Build history of the part. All positions in model axes, mm. A direction names the side the tool comes from. Give positions to 0.01 mm unless a question says otherwise; leave off trailing zeros. Order: outer loops, then holes, each group sorted by start corner. A loop starts at its lowest first (then second) coordinate and runs counter-clockwise, first axis right, second up. Notation, with made-up numbers: (54.5, 87) - (72.5, 87) arc R9 ccw to (72.5, 92) - close; hole circle Ø2 at (1.5, 15). An arc over 180 degrees is marked (long way). Write each question's results on one line, items separated by ' | '. Start each with the question number.
1) Two-plate mould, pull along Y, no slides. Class faces 4 (the face through (0, 46.189, 1)), 5 (the face through (21.09, -36.31, 68.49)), 6 (the face through (0, -26.707, 16)): +Y half, -Y half, draft (parallel to the pull), parting line (faces both ways), or undercut.
2) Tool access for faces 1 (the face through (-21.18, 0.59, -26.29)), 2 (the face through (21.18, 0.59, -26.29)), 3 (the face through (29.472, 37, -1)): list every direction of +Z, -Z, +X, -X, +Y, -Y with a clear straight run to the whole face (end or side of a thin tool).
3) Drop flat-ended pins along their axis: pin 1 Ø10 at (x, y) = (-6, -33) entering from -Z; pin 2 Ø4 at (x, y) = (-19.5, 24) entering from -Z; pin 3 Ø5 at (x, y) = (7.5, 2.5) entering from -Z. Give the stop position or say it passes through.
4) Drill centre lines: line 1 along Y through (x, z) = (-25, 37); line 2 along Z through (x, y) = (-3.5, -29); line 3 along Z through (x, y) = (-7, -34). Where is each one in solid material? Low to high. Write a range as from..to.
5) Cut at C-C on z = 59. List the corners of the cut face in (x, y).
6) Cut at A-A on y = 33. List the corners of the cut face in (x, z).
7) Cut at D-D on x = -7.5. List the corners of the cut face in (y, z).
8) Cut at B-B on z = -9.5. List the corners of the cut face in (x, y).
from build123d import *

# Parameters (mm, degrees)
F0_W        = 58.9435696602
F0_H        = 155.2014648914
F4_DEPTH    = 46.1890073493
F5_W        = 53.8340881467
F5_H        = 92.8563177586
F1_DEPTH    = 58.9445696602
F2_T1_DEPTH = 168.3050352459
F2_T3_DEPTH = 168.726075006
F2_T5_DEPTH = 241.6216065486
F3_T1_DEPTH = 53.8340881467
F6_R        = 13.164421927
F6_R_2      = 14.3764863779
F7_DEPTH    = 92.3790146986


# Not quite as in the source:
# - a fillet or chamfer that OpenCascade refuses, or shapes differently, is made with other operations: its cross-section is extruded or revolved along the edge and cut away or added


with BuildPart() as f4:
    # F0 (on Front) → F4 (new body, symmetric)
    with BuildSketch(Plane.XZ):
        Rectangle(F0_W, F0_H)
    extrude(amount=F4_DEPTH, both=True)

    # F5 (on face) → F1 (cut, through all)
    with BuildSketch(Plane.YZ.offset(29.4717848301)):
        with Locations((0.2105198801, 31.1725735664)):
            Rectangle(F5_W, F5_H)
    extrude(amount=-F1_DEPTH, mode=Mode.SUBTRACT)

    # F2: fillet of radius 29.84871837 on 6 edges, made by hand

    # F2_s2 → F2_t1 (cut)
    with BuildSketch(Plane.XZ.offset(-120.8108032743)):
        with BuildLine():
            ThreePointArc((29.4717848301, 47.7520140757), (20.7292976292, 68.8582452449), (-0.3769335399, 77.6007324457))
            Line((-0.3769335399, 77.6007324457), (29.4717848301, 77.6007324457))
            Line((29.4717848301, 77.6007324457), (29.4717848301, 47.7520140757))
        make_face()
        with BuildLine():
            ThreePointArc((-29.4717848301, 47.7520140757), (-20.7292976292, 68.8582452449), (0.3769335399, 77.6007324457))
            Line((0.3769335399, 77.6007324457), (-29.4717848301, 77.6007324457))
            Line((-29.4717848301, 77.6007324457), (-29.4717848301, 47.7520140757))
        make_face()
    extrude(amount=F2_T1_DEPTH, mode=Mode.SUBTRACT)

    # F2_s4 → F2_t3 (cut)
    with BuildSketch(Plane.XZ.offset(-47.9152717317)):
        with BuildLine():
            ThreePointArc((29.4717848301, 47.7520140757), (20.7292976292, 68.8582452449), (-0.3769335399, 77.6007324457))
            Line((-0.3769335399, 77.6007324457), (29.4717848301, 77.6007324457))
            Line((29.4717848301, 77.6007324457), (29.4717848301, 47.7520140757))
        make_face()
        with BuildLine():
            ThreePointArc((-29.4717848301, 47.7520140757), (-20.7292976292, 68.8582452449), (0.3769335399, 77.6007324457))
            Line((0.3769335399, 77.6007324457), (-29.4717848301, 77.6007324457))
            Line((-29.4717848301, 77.6007324457), (-29.4717848301, 47.7520140757))
        make_face()
    extrude(amount=F2_T3_DEPTH, mode=Mode.SUBTRACT)

    # F2_s6 → F2_t5 (cut)
    with BuildSketch(Plane.XZ.offset(-120.8108032743)):
        with BuildLine():
            ThreePointArc((-0.3769335399, -77.6007324457), (20.7292976292, -68.8582452449), (29.4717848301, -47.7520140757))
            Line((29.4717848301, -47.7520140757), (29.4717848301, -77.6007324457))
            Line((29.4717848301, -77.6007324457), (-0.3769335399, -77.6007324457))
        make_face()
        with BuildLine():
            ThreePointArc((0.3769335399, -77.6007324457), (-20.7292976292, -68.8582452449), (-29.4717848301, -47.7520140757))
            Line((-29.4717848301, -47.7520140757), (-29.4717848301, -77.6007324457))
            Line((-29.4717848301, -77.6007324457), (0.3769335399, -77.6007324457))
        make_face()
    extrude(amount=F2_T5_DEPTH, mode=Mode.SUBTRACT)

    # F3: fillet of radius 32.8509948239 on 2 edges, made by hand

    # F3_s2 → F3_t1 (cut)
    with BuildSketch(Plane.XZ.offset(-27.1275639534)):
        with BuildLine():
            ThreePointArc((29.4717848301, -48.1065801367), (19.8499512149, -24.877418928), (-3.3792099938, -15.2555853128))
            Line((-3.3792099938, -15.2555853128), (29.4717848301, -15.2555853128))
            Line((29.4717848301, -15.2555853128), (29.4717848301, -48.1065801367))
        make_face()
        with BuildLine():
            ThreePointArc((-29.4717848301, -48.1065801367), (-19.8499512149, -24.877418928), (3.3792099938, -15.2555853128))
            Line((3.3792099938, -15.2555853128), (-29.4717848301, -15.2555853128))
            Line((-29.4717848301, -15.2555853128), (-29.4717848301, -48.1065801367))
        make_face()
    extrude(amount=F3_T1_DEPTH, mode=Mode.SUBTRACT)

    # F6 (on face) → F7 (cut, through all)
    with BuildSketch(Plane.XZ.offset(46.1890073493)):
        with Locations((0.3769335399, 47.7520140757)):
            Circle(F6_R)
        with Locations((0.3769335399, -47.7520140757)):
            Circle(F6_R_2)
    extrude(amount=-F7_DEPTH, mode=Mode.SUBTRACT)


solid = f4.part
Results:
1) face 4: +Y half | face 5: draft | face 6: undercut
2) face 1: +Z, -X | face 2: +Z, +X | face 3: +Z, -Z, +X, +Y, -Y
3) pin 1: z = -77.57 | pin 2: z = -71.66 | pin 3: z = -77.11
4) line 1: -46.19..-26.71, 27.13..46.19 | line 2: -77.35..-61.6, -33.91..35.17, 60.33..77.35 | line 3: -76.67..-60.09, -35.41..36.85, 58.66..76.67
5) outline: (-27.27, -46.19) - (-6.46, -46.19) - (-6.46, -26.71) - (-27.27, -26.71) - close; (-27.27, 27.13) - (-6.46, 27.13) - (-6.46, 46.19) - (-27.27, 46.19) - close; (7.22, -46.19) - (27.27, -46.19) - (27.27, -26.71) - (7.22, -26.71) - close; (7.22, 27.13) - (27.27, 27.13) - (27.27, 46.19) - (7.22, 46.19) - close
6) outline: (-29.47, -47.75) arc R29.85 ccw to (0, -77.6) arc R29.85 ccw to (29.47, -47.75) - (29.47, 47.75) arc R29.85 ccw to (0, 77.6) arc R29.85 ccw to (-29.47, 47.75) - close; hole circle Ø28.75 at (0.38, -47.75); hole circle Ø26.33 at (0.38, 47.75)
7) outline: (-46.19, -76.54) - (46.19, -76.54) - (46.19, -59.78) - (-46.19, -59.78) - close; (-46.19, -35.73) - (46.19, -35.73) - (46.19, 37.2) - (27.13, 37.2) - (27.13, -17.11) - (-26.71, -17.11) - (-26.71, 37.2) - (-46.19, 37.2) - close; (-46.19, 58.3) - (-26.71, 58.3) - (-26.71, 76.54) - (-46.19, 76.54) - close; (27.13, 58.3) - (46.19, 58.3) - (46.19, 76.54) - (27.13, 76.54) - close
8) outline: (-29.47, -46.19) - (29.47, -46.19) - (29.47, -26.71) - (-29.47, -26.71) - close; (-29.47, 27.13) - (29.47, 27.13) - (29.47, 46.19) - (-29.47, 46.19) - close
